CAD build for the part. Positions are in the model's coordinates, mm. A direction names the side the tool comes from. Coordinates: 2 decimals unless noted, no trailing zeros. Loops run counter-clockwise (first coordinate to the right, second up) from the corner with the lowest first, then second, coordinate; pieces in that order, holes last. Notation, with made-up numbers: (25, -28.5) -> (29, -28.5) arc R24 ccw to (29, -15.5) -> close; hole circle Ø8 at (-22.75, 56.25). An arc over 180 degrees is marked (long way). Return JSON: item names as keys, results as strings. Group by question number.
(1) Saw through at A-A on y = 0. Write the cut outline in (x, z), then the cut area to 3 significant figures.
(2) Saw through at C-C on x = -15. Write the cut outline in (y, z), then the cut area to 3 significant figures.
(3) Flat gauge pins, fed straight in: pin 1 Ø10 at (x, y) = (-1.5, 12) entering from -Z; pin 2 Ø3 at (y, z) = (7.75, 13.42) entering from +X; pin 3 Ø5 at (x, z) = (2, 13) entering from -Y. Where does each tip first touch, or does it go through?
(4) Tool access for faces 5 (the face through (-6.5, -0.1, 3.7)), 6 (the face through (60.577, -6.083, -6.633)), 7 (the face through (-22, 0, 7)): list every direction of +Z, -Z, +X, -X, +Y, -Y with a clear straight run to the whole face (end or side of a thin tool).
(5) Mould opens along Y. For faces 1 (the face through (7.605, 16.554, -0.672)), 2 (the face through (25, 14.9, -9.5)), 3 (the face through (-16, -2.4, 7)), 4 (the face through (12.3, 11.2, -14.6)) say: pulls with the +Y half, pulls with the -Y half, needs draft (parallel to the pull), parting line crosses it, or undercut.
(6) Saw through at B-B on x = 14. Write the cut outline in (y, z).
(7) Saw through at D-D on z = 15.5. Write the cut outline in (x, y).
(8) Probe L1, parallel to Y at x = 9, z = 0; L2, parallel to X at y = -9, z = 14; L3, parallel to X at y = -7, z = 3. List the from-to ranges inside material, lowest first.
```python
from build123d import *

# Parameters (mm, degrees)
ESQUISSE3_W                                   = 15.5
ESQUISSE3_H                                   = 3
ESQUISSE3_W_2                                 = 6.5
ESQUISSE3_H_2                                 = 6
CHANFREIN1_SIZE                               = 1
ENL_V_MAT_EXTRU_1_DEPTH                       = 82.278041315
ENL_V_MAT_EXTRU_1_DEPTH_BACK                  = 12
TROU_POUR_TARAUDAGE_POUR_TROU_TARAUD_M3_D     = 2.5
TROU_POUR_TARAUDAGE_POUR_TROU_TARAUD_M3_DEPTH = 15
TROU_POUR_TARAUDAGE_POUR_TROU_TARAUD_M3_TIP   = 0.751075774
ESQUISSE9_W                                   = 11
ESQUISSE9_H                                   = 9


with BuildPart() as part:
    # Esquisse1 → Révolution10 (revolve)
    with BuildSketch(Plane.XY, mode=Mode.PRIVATE) as r_volution10_sk:
        Polygon((0, 6), (0, 0), (12.5, 0), (55, 0), (55, 17.5), (25, 17.5), (25, 18.4), (0, 18.4), align=None)
    revolve(r_volution10_sk.sketch.rotate(Axis((12.5, 0, 0), (1, 0, 0)), 90), axis=Axis((12.5, 0, 0), (1, 0, 0)))

    # Esquisse3 → Révolution12 (revolve)
    with BuildSketch(Plane.XY.offset(7), mode=Mode.PRIVATE) as r_volution12_sk:
        with Locations((-14.25, 1.5)):
            Rectangle(ESQUISSE3_W, ESQUISSE3_H)
        with Locations((-3.25, 3)):
            Rectangle(ESQUISSE3_W_2, ESQUISSE3_H_2)
    revolve(r_volution12_sk.sketch.rotate(Axis((0, 0, 7), (1, 0, 0)), 90), axis=Axis((0, 0, 7), (1, 0, 0)))

    # Chanfrein1
    chanfrein1_edges = [part.edges().sort_by_distance(p)[0] for p in [
        (-6.5, 0, 1),
    ]]
    chamfer(chanfrein1_edges, length=CHANFREIN1_SIZE)

    # Esquisse4 → Enlèv. mat.-Extru.1 (cut, two sides: drawn at the far end of the back side and taken through both)
    with BuildSketch(Plane.ZY.offset(22).offset(-ENL_V_MAT_EXTRU_1_DEPTH_BACK)):
        Polygon((-73.282990589, -2.4), (5.2, -2.4), (8.8, -2.4), (87.282990589, -2.4), (87.282990589, -159.365981178), (-73.282990589, -159.365981178), align=None)
    extrude(amount=ENL_V_MAT_EXTRU_1_DEPTH + ENL_V_MAT_EXTRU_1_DEPTH_BACK, mode=Mode.SUBTRACT)

    # Trou pour taraudage pour trou taraudé M3x0.51
    with Locations(Plane.ZY):
        with Locations((0, 15.5), (-13.423393759, -7.75), (0, -15.5), (13.423393759, -7.75), (13.423393759, 7.75), (-13.423393759, 7.75)):
            Hole(TROU_POUR_TARAUDAGE_POUR_TROU_TARAUD_M3_D / 2, depth=TROU_POUR_TARAUDAGE_POUR_TROU_TARAUD_M3_DEPTH)
            with Locations((0, 0, -(TROU_POUR_TARAUDAGE_POUR_TROU_TARAUD_M3_DEPTH + TROU_POUR_TARAUDAGE_POUR_TROU_TARAUD_M3_TIP / 2))):  # 118° drill point
                Cone(0, TROU_POUR_TARAUDAGE_POUR_TROU_TARAUD_M3_D / 2, TROU_POUR_TARAUDAGE_POUR_TROU_TARAUD_M3_TIP, mode=Mode.SUBTRACT)

    # Esquisse9 → Révolution13 (revolve)
    with BuildSketch(Plane.XY, mode=Mode.PRIVATE) as r_volution13_sk:
        with Locations((60.5, 4.5)):
            Rectangle(ESQUISSE9_W, ESQUISSE9_H)
    revolve(r_volution13_sk.sketch.rotate(Axis((0, 0, 0), (1, 0, 0)), 90), axis=Axis((0, 0, 0), (1, 0, 0)))


solid = part.part
```
Geometry results:
{
 "1": {"outline": "(-22, 4) -> (-6.5, 4) -> (-6.5, 2) -> (-5.5, 1) -> (0, 1) -> (0, -18.4) -> (25, -18.4) -> (25, -17.5) -> (55, -17.5) -> (55, -9) -> (66, -9) -> (66, 9) -> (55, 9) -> (55, 17.5) -> (25, 17.5) -> (25, 18.4) -> (0, 18.4) -> (0, 13) -> (-5.5, 13) -> (-6.5, 12) -> (-6.5, 10) -> (-22, 10) -> close", "area": "2,340 mm²"},
 "2": {"outline": "(-2.4, 5.2) arc R3 ccw (long way) to (-2.4, 8.8) -> close", "area": "26.8 mm²"},
 "3": {"pin 1": "z = -16.92", "pin 2": "x = 55", "pin 3": "y = -15.11"},
 "4": {"face 5": "-X", "face 6": "+X", "face 7": "+Z, -Z, -X, +Y, -Y"},
 "5": {"face 1": "undercut", "face 2": "needs draft", "face 3": "pulls with the -Y half", "face 4": "parting line crosses it"},
 "6": {"outline": "circle Ø36.8 at (0, 0); hole circle Ø2.5 at (-15.5, 0); hole circle Ø2.5 at (-7.75, -13.42); hole circle Ø2.5 at (-7.75, 13.42); hole circle Ø2.5 at (7.75, -13.42); hole circle Ø2.5 at (7.75, 13.42); hole circle Ø2.5 at (15.5, 0)"},
 "7": {"outline": "(0, -9.92) -> (25, -9.92) -> (25, -8.12) -> (55, -8.12) -> (55, 8.12) -> (25, 8.12) -> (25, 9.92) -> (0, 9.92) -> close"},
 "8": {"L1": "-18.4 to -16.75, -14.25 to 14.25, 16.75 to 18.4", "L2": "0 to 55", "L3": "0 to 66"}
}
